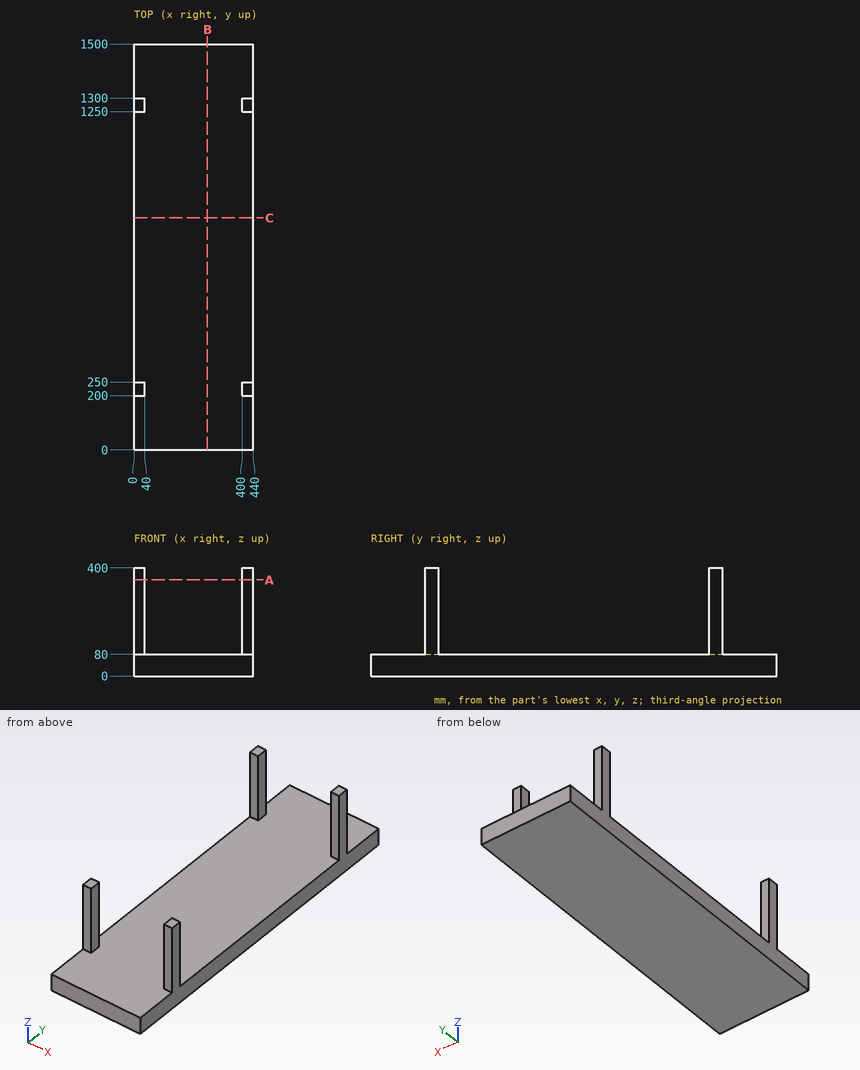
Could you check a few things on this drawing? It's one solid part, dimensions in mm from its lowest x, y, z. Give positions to 0.01 mm unless a question says otherwise; leave off trailing zeros. Loops run counter-clockwise (first coordinate to the right, second up) from the corner with the lowest first, then second, coordinate; pieces in that order, holes last. Notation, with made-up numbers: M 66,69.5 L 110,69.5 A18 ccw 110,78.5 Z; hole C -5,80.25 d7. An arc over 180 degrees is marked long. Answer as a JSON object with one key per item and string values.
Q1. Suppose I cut it at A-A, the plane z = 355.5. List the corners of the cut face in (x, y) for me, plus the area to 3 significant figures.
Values found:
{"outline": "M 0,200 L 40,200 L 40,250 L 0,250 Z; M 0,1250 L 40,1250 L 40,1300 L 0,1300 Z; M 400,200 L 440,200 L 440,250 L 400,250 Z; M 400,1250 L 440,1250 L 440,1300 L 400,1300 Z", "area": "8,000 mm²"}
Q2. Suppose I cut it at C-C, the plane y = 857.5. List the corners of the cut face in (x, z) for me, plus the area to 3 significant figures.
Values found:
{"outline": "M 0,0 L 440,0 L 440,80 L 0,80 Z", "area": "35,200 mm²"}
Q3. If I drill on probe 1 along X at (y, z) = (207, 257); probe 2 along Y at (x, z) = (34.5, 371.5); probe 3 along Z at (x, y) = (183, 850), over which ranges is the centre line in solid material (lowest first)? Write a range as [from, to].
Values found:
{"probe 1": "x = [0, 40], [400, 440]", "probe 2": "y = [200, 250], [1250, 1300]", "probe 3": "z = [0, 80]"}
Q4. Suppose I cut it at B-B, the plane x = 270.5. List the corners of the cut face in (y, z) for me.
Values found:
{"outline": "M 0,0 L 1500,0 L 1500,80 L 0,80 Z"}
Q5. For P1, Ø12, axis at x = 390.5, y = 422.5, coming from the +Z side; P2, Ø20, axis at x = 11, z = 283, coming from the -Y side; P3, Ø12, axis at x = 415, z = 264, coming from the +Y side, each with a flat end and sliding along its axis, tell me the tip position at first contact or that it passes through.
Values found:
{"P1": "stops at z = 80", "P2": "stops at y = 200", "P3": "stops at y = 1300"}
